Build history of the part. All positions in model axes, mm. Face numbers are marked on the shaded views. A direction names the side the tool comes from. Round coordinates to 2 decimals unless told otherwise and drop trailing zeros. Loops run counter-clockwise (first coordinate to the right, second up) from the corner with the lowest first, then second, coordinate; pieces in that order, holes last. Notation, with made-up numbers: M -10.75,-23.75 L 43.25,-23.75 A23 ccw 43.25,-2.75 Z; hole C 10.5,62 d9. An arc over 180 degrees is marked long. Use one line per item in the form item = value. Start each with the question number.
```python
from build123d import *

# Parameters (mm, degrees)
SKETCH1_W               = 200
SKETCH1_H               = 95
SKETCH1_R               = 1.75
BOSS_EXTRUDE1_DEPTH     = 5
SKETCH2_R               = 15
SKETCH2_R_2             = 12.5
CUT_EXTRUDE1_DEPTH      = 5
SKETCH4_W               = 16
SKETCH4_H               = 37
BOSS_EXTRUDE2_DEPTH     = 4.2
SKETCH6_W               = 20
SKETCH6_H               = 95
BOSS_EXTRUDE3_DEPTH     = 3
BOSS_EXTRUDE4_START     = 4
BOSS_EXTRUDE4_DEPTH     = 4
SKETCH9_R               = 13
BOSS_EXTRUDE5_DEPTH     = 2
CUT_EXTRUDE2_DEPTH      = 5
SKETCH11_R              = 1.75
CUT_EXTRUDE3_DEPTH      = 10
CUT_EXTRUDE4_DEPTH      = 10
CUT_EXTRUDE4_DEPTH_BACK = 10
SKETCH14_R              = 1.75


with BuildPart() as part:
    # Sketch1 → Boss-Extrude1 (new body)
    with BuildSketch(Plane(origin=(0, 0, 0), x_dir=(1, 0, 0), z_dir=(0, 1, 0))):
        Rectangle(SKETCH1_W, SKETCH1_H)
        with Locations(Location((-96, 43.5, 0), (0, 0, 270))):
            Circle(SKETCH1_R, mode=Mode.SUBTRACT)
        with Locations(Location((-96, -43.5, 0), (0, 0, 270))):
            Circle(SKETCH1_R, mode=Mode.SUBTRACT)
        with Locations(Location((97, 43.5, 0), (0, 0, 270))):
            Circle(SKETCH1_R, mode=Mode.SUBTRACT)
        with Locations(Location((97, -43.5, 0), (0, 0, 270))):
            Circle(SKETCH1_R, mode=Mode.SUBTRACT)
    extrude(amount=BOSS_EXTRUDE1_DEPTH)

    # Sketch2 → Cut-Extrude1 (cut)
    with BuildSketch(Plane(origin=(0, 5, 0), x_dir=(1, 0, 0), z_dir=(0, 1, 0))):
        with Locations((33.5, 0)):
            Circle(SKETCH2_R)
        with BuildLine():
            ThreePointArc((48.5, 0), (39.240251485, -13.858192988), (22.893398282, -10.606601718))
            Line((22.893398282, -10.606601718), (47.393398282, -35.106601718))
            ThreePointArc((47.393398282, -35.106601718), (52.259748515, -10.641807012), (73, -24.5))
            ThreePointArc((73, -24.5), (71.858192988, -30.240251485), (68.606601718, -35.106601718))
            Line((68.606601718, -35.106601718), (93.106601718, -10.606601718))
            ThreePointArc((93.106601718, -10.606601718), (67.5, 0), (93.106601718, 10.606601718))
            Line((93.106601718, 10.606601718), (68.606601718, 35.106601718))
            ThreePointArc((68.606601718, 35.106601718), (71.858192988, 30.240251485), (73, 24.5))
            ThreePointArc((73, 24.5), (52.259748515, 10.641807012), (47.393398282, 35.106601718))
            Line((47.393398282, 35.106601718), (22.893398282, 10.606601718))
            ThreePointArc((22.893398282, 10.606601718), (39.240251485, 13.858192988), (48.5, 0))
        make_face()
        with Locations((58, -24.5)):
            Circle(SKETCH2_R)
        with Locations((82.5, 0)):
            Circle(SKETCH2_R)
        with Locations((58, 24.5)):
            Circle(SKETCH2_R)
        with Locations(Location((-82, -27.5, 0), (0, 0, 270))):
            Circle(SKETCH2_R_2)
    extrude(amount=-CUT_EXTRUDE1_DEPTH, mode=Mode.SUBTRACT)

    # Sketch4 → Boss-Extrude2 (add)
    with BuildSketch(Plane.XZ):
        with Locations((-82.5, -19.5)):
            Rectangle(SKETCH4_W, SKETCH4_H)
    extrude(amount=BOSS_EXTRUDE2_DEPTH)

    # Sketch6 → Boss-Extrude3 (add)
    with BuildSketch(Plane(origin=(0, 5, 0), x_dir=(1, 0, 0), z_dir=(0, 1, 0))):
        with Locations((-110, 0)):
            Rectangle(SKETCH6_W, SKETCH6_H)
        with Locations((110, 0)):
            Rectangle(SKETCH6_W, SKETCH6_H)
    extrude(amount=-BOSS_EXTRUDE3_DEPTH)

    # Sketch8 → Boss-Extrude4 (add)
    with BuildSketch(Plane(origin=(0, 5, 0), x_dir=(1, 0, 0), z_dir=(0, 1, 0)).offset(BOSS_EXTRUDE4_START)):
        with BuildLine():
            Line((70.727922061, -37.227922061), (95.227922061, -12.727922061))
            ThreePointArc((95.227922061, -12.727922061), (100.5, 0), (95.227922061, 12.727922061))
            Line((95.227922061, 12.727922061), (70.727922061, 37.227922061))
            ThreePointArc((70.727922061, 37.227922061), (58, 42.5), (45.272077939, 37.227922061))
            Line((45.272077939, 37.227922061), (20.772077939, 12.727922061))
            ThreePointArc((20.772077939, 12.727922061), (15.5, 0), (20.772077939, -12.727922061))
            Line((20.772077939, -12.727922061), (45.272077939, -37.227922061))
            ThreePointArc((45.272077939, -37.227922061), (58, -42.5), (70.727922061, -37.227922061))
        make_face()
        with BuildLine():
            Line((22.893398282, -10.606601718), (47.393398282, -35.106601718))
            ThreePointArc((47.393398282, -35.106601718), (58, -39.5), (68.606601718, -35.106601718))
            Line((68.606601718, -35.106601718), (93.106601718, -10.606601718))
            ThreePointArc((93.106601718, -10.606601718), (97.5, 0), (93.106601718, 10.606601718))
            Line((93.106601718, 10.606601718), (68.606601718, 35.106601718))
            ThreePointArc((68.606601718, 35.106601718), (58, 39.5), (47.393398282, 35.106601718))
            Line((47.393398282, 35.106601718), (22.893398282, 10.606601718))
            ThreePointArc((22.893398282, 10.606601718), (18.5, 0), (22.893398282, -10.606601718))
        make_face(mode=Mode.SUBTRACT)
    extrude(amount=-BOSS_EXTRUDE4_DEPTH)

    # Sketch9 → Boss-Extrude5 (add)
    with BuildSketch(Plane(origin=(0, 9, 0), x_dir=(1, 0, 0), z_dir=(0, 1, 0))):
        with BuildLine():
            Line((22.893398282, -10.606601718), (47.393398282, -35.106601718))
            ThreePointArc((47.393398282, -35.106601718), (58, -39.5), (68.606601718, -35.106601718))
            Line((68.606601718, -35.106601718), (93.106601718, -10.606601718))
            ThreePointArc((93.106601718, -10.606601718), (97.5, 0), (93.106601718, 10.606601718))
            Line((93.106601718, 10.606601718), (68.606601718, 35.106601718))
            ThreePointArc((68.606601718, 35.106601718), (58, 39.5), (47.393398282, 35.106601718))
            Line((47.393398282, 35.106601718), (22.893398282, 10.606601718))
            ThreePointArc((22.893398282, 10.606601718), (18.5, 0), (22.893398282, -10.606601718))
        make_face()
        with Locations(Location((58, 24.5, 0), (0, 0, 270))):
            Circle(SKETCH9_R, mode=Mode.SUBTRACT)
        with Locations(Location((82.5, 0, 0), (0, 0, 270))):
            Circle(SKETCH9_R, mode=Mode.SUBTRACT)
        with Locations(Location((58, -24.5, 0), (0, 0, 270))):
            Circle(SKETCH9_R, mode=Mode.SUBTRACT)
        with Locations(Location((33.5, 0, 0), (0, 0, 270))):
            Circle(SKETCH9_R, mode=Mode.SUBTRACT)
    extrude(amount=-BOSS_EXTRUDE5_DEPTH)

    # Sketch10 → Cut-Extrude2 (cut)
    with BuildSketch(Plane(origin=(0, 5, 0), x_dir=(1, 0, 0), z_dir=(0, 1, 0))):
        Polygon((0, 38.5), (-7.778174593, 30.721825407), (0, 22.943650814), (7.778174593, 30.721825407), align=None)
    extrude(amount=-CUT_EXTRUDE2_DEPTH, mode=Mode.SUBTRACT)

    # Sketch11 → Cut-Extrude3 (cut)
    with BuildSketch(Plane(origin=(0, 5, 0), x_dir=(1, 0, 0), z_dir=(0, 1, 0))):
        with Locations(Location((-35.721825407, 43.5, 0), (0, 0, 270))):
            Circle(SKETCH11_R)
        with Locations(Location((-25.721825407, 43.5, 0), (0, 0, 270))):
            Circle(SKETCH11_R)
        with Locations(Location((5, -43.5, 0), (0, 0, 270))):
            Circle(SKETCH11_R)
        with Locations(Location((-5, -43.5, 0), (0, 0, 270))):
            Circle(SKETCH11_R)
    extrude(amount=-CUT_EXTRUDE3_DEPTH, mode=Mode.SUBTRACT)

    # Sketch14 → Cut-Extrude4 (cut, two sides: drawn at the far end of the back side and taken through both)
    # profile 1 of 3: a face of its own
    with BuildSketch(Plane(origin=(0, 5, 0), x_dir=(1, 0, 0), z_dir=(0, 1, 0)).offset(-CUT_EXTRUDE4_DEPTH_BACK)):
        Polygon((-30.721825407, 47.5), (-30.721825407, 30.721825407), (0, 0), (0, -47.5), (120, -47.5), (120, 47.5), align=None)
        with Locations((5, -43.5)):
            Circle(SKETCH14_R, mode=Mode.SUBTRACT)
        with Locations((97, -43.5)):
            Circle(SKETCH14_R, mode=Mode.SUBTRACT)
        with BuildLine():
            ThreePointArc((45.272077939, 37.227922061), (58, 42.5), (70.727922061, 37.227922061))
            Line((70.727922061, 37.227922061), (95.227922061, 12.727922061))
            ThreePointArc((95.227922061, 12.727922061), (100.5, 0), (95.227922061, -12.727922061))
            Line((95.227922061, -12.727922061), (70.727922061, -37.227922061))
            ThreePointArc((70.727922061, -37.227922061), (58, -42.5), (45.272077939, -37.227922061))
            Line((45.272077939, -37.227922061), (20.772077939, -12.727922061))
            ThreePointArc((20.772077939, -12.727922061), (15.5, 0), (20.772077939, 12.727922061))
            Line((20.772077939, 12.727922061), (45.272077939, 37.227922061))
        make_face(mode=Mode.SUBTRACT)
        with Locations((-25.721825407, 43.5)):
            Circle(SKETCH14_R, mode=Mode.SUBTRACT)
        Polygon((-7.778174593, 30.721825407), (0, 38.5), (7.778174593, 30.721825407), (0, 22.943650814), align=None, mode=Mode.SUBTRACT)
        with Locations((97, 43.5)):
            Circle(SKETCH14_R, mode=Mode.SUBTRACT)
    # profile 2 of 3: a face of its own
    with BuildSketch(Plane(origin=(0, 5, 0), x_dir=(1, 0, 0), z_dir=(0, 1, 0)).offset(-CUT_EXTRUDE4_DEPTH_BACK)):
        with BuildLine():
            Line((70.727922061, 37.227922061), (95.227922061, 12.727922061))
            ThreePointArc((95.227922061, 12.727922061), (100.5, 0), (95.227922061, -12.727922061))
            Line((95.227922061, -12.727922061), (70.727922061, -37.227922061))
            ThreePointArc((70.727922061, -37.227922061), (58, -42.5), (45.272077939, -37.227922061))
            Line((45.272077939, -37.227922061), (20.772077939, -12.727922061))
            ThreePointArc((20.772077939, -12.727922061), (15.5, 0), (20.772077939, 12.727922061))
            Line((20.772077939, 12.727922061), (45.272077939, 37.227922061))
            ThreePointArc((45.272077939, 37.227922061), (58, 42.5), (70.727922061, 37.227922061))
        make_face()
    # profile 3 of 3: a face of its own
    with BuildSketch(Plane(origin=(0, 5, 0), x_dir=(1, 0, 0), z_dir=(0, 1, 0)).offset(-CUT_EXTRUDE4_DEPTH_BACK)):
        Polygon((0, 38.5), (7.778174593, 30.721825407), (0, 22.943650814), (-7.778174593, 30.721825407), align=None)
    extrude(amount=CUT_EXTRUDE4_DEPTH + CUT_EXTRUDE4_DEPTH_BACK, mode=Mode.SUBTRACT)


solid = part.part
```
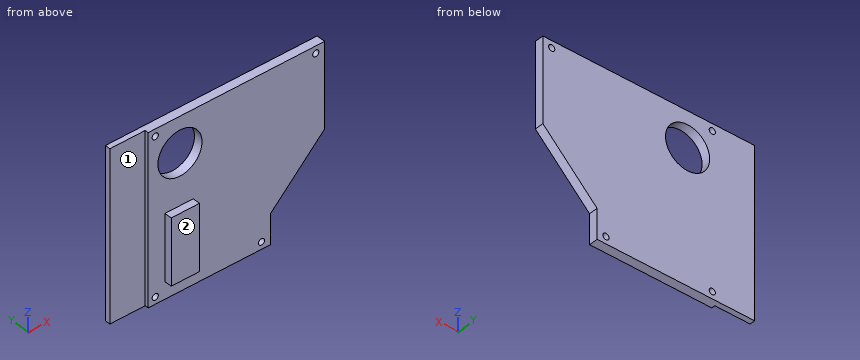
Q1. Drop flat-ended pins along their axis: P1, Ø1.3, axis at y = -3, z = -26.5, coming from the +X side; P2, Ø4, axis at x = -5, z = 43.5, coming from the -Y side; P3, Ø5.5, axis at y = 1.5, z = -37, coming from the +X side. Give the stop position or say it passes through.
Q2. Saw through at D-D (y = -2.5). Give the cut face in (x, z), and give its area (3 significant figures).
Q3. Saw through at B-B (x = -92). Give the cut face in (y, z), and give its area (3 significant figures).
Q4. Saw through at A-A (z = 27.5). Give the cut face in (x, y), and give its area (3 significant figures).
Q5. Tool access for the marked faces 1 and 2: list every direction of +Z, -Z, +X, -X, +Y, -Y with a clear straight run to the whole face (end or side of a thin tool).
Q6. Saw through at C-C (z = -43.5). Give the cut face in (x, y).
Q7. Wall check: probe 1 along Z at (x, y) = (-96, 1.25); probe 2 along X at (y, z) = (1.7, 27.5); probe 3 along Y at (x, z) = (-51.5, -41). Give the ranges that are in metal, low to high.
Filled in:
q1.P1 = -74.5
q1.P2 = 0
q1.P3 = -30.72
q2.outline = M -90.5,-38 L -74.5,-38 L -74.5,-1 L -90.5,-1 Z
q2.area = 592 mm²
q3.outline = M 0,-47.5 L 5,-47.5 L 5,20 L 0,20 Z; M 0,35 L 5,35 L 5,47.5 L 0,47.5 Z
q3.area = 400 mm²
q4.outline = M -120,2 L -100,2 L -100,0 L -94.5,0 L -94.5,5 L -120,5 Z; M -69.5,0 L 0,0 L 0,5 L -69.5,5 Z
q4.area = 435 mm²
q5.face_1 = +Z, -Z, -X, -Y
q5.face_2 = +Z, -Z, +X, -X, -Y
q6.outline = M -120,2 L -100,2 L -100,0 L -97.75,0 L -97.75,5 L -120,5 Z; M -94.25,0 L -37.47,0 L -37.47,5 L -94.25,5 Z; M -33.97,0 L -30.72,0 L -30.72,5 L -33.97,5 Z
q7.probe_1 = -47.5 to -45.25, -41.75 to 41.75, 45.25 to 47.5
q7.probe_2 = -100 to -94.5, -69.5 to 0
q7.probe_3 = 0 to 5
